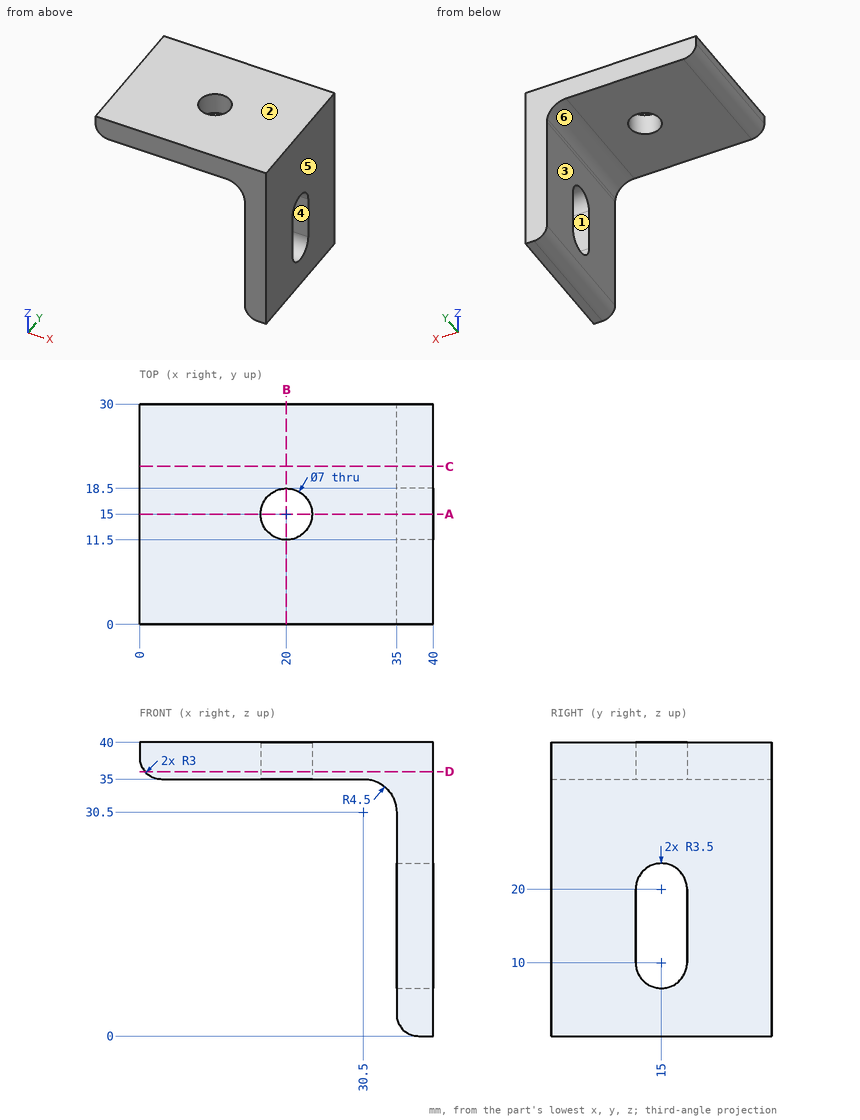
The figure shows three views and two pictorial views of one solid part (mm, origin at its lowest corner). Answer the questions. A direction names the side the tool comes from. Give positions to 0.01 mm unless a question says otherwise; leave off trailing zeros. Order: outer loops, then holes, each group sorted by start corner. A loop starts at its lowest first (then second) coordinate and runs counter-clockwise, first axis right, second up. Notation, with made-up numbers: (57, 13.5) -> (75, 13.5) arc R17 cw to (75, 43.5) -> close; hole circle Ø6 at (34.5, 75). An arc over 180 degrees is marked (long way). One line per item, written item: value.
1) Find section A-A, the plane y = 15. Determine the outline of the cut face in (x, z).
Reported:
outline: (0, 38) arc R3 ccw to (3, 35) -> (16.5, 35) -> (16.5, 40) -> (0, 40) -> close; (23.5, 35) -> (30.5, 35) arc R4.5 cw to (34.93, 31.3) arc R4.5 cw to (35, 30.5) -> (35, 23.5) -> (40, 23.5) -> (40, 40) -> (23.5, 40) -> close; (35, 3) arc R3 ccw to (38, 0) -> (40, 0) -> (40, 6.5) -> (35, 6.5) -> close
2) Find section D-D, the plane z = 36. Determine the outline of the cut face in (x, y), plus the area to 3 significant figures.
Reported:
outline: (0.76, 0) -> (40, 0) -> (40, 30) -> (0.76, 30) -> close; hole circle Ø7 at (20, 15)
area: 1,140 mm^2
3) Determine the mould class of the marked faces 4, 5 and 6 for opening direction Z: pulls with the +Z half, pulls with the -Z half, needs draft (parallel to the pull), parting line crosses it, or undercut.
Reported:
face 4: undercut
face 5: needs draft
face 6: pulls with the -Z half
4) Find section B-B, the plane x = 20. Determine the outline of the cut face in (y, z), plus the area to 3 significant figures.
Reported:
outline: (0, 35) -> (11.5, 35) -> (11.5, 40) -> (0, 40) -> close; (18.5, 35) -> (30, 35) -> (30, 40) -> (18.5, 40) -> close
area: 115 mm^2
5) Find section C-C, the plane y = 21.5. Determine the outline of the cut face in (x, z).
Reported:
outline: (0, 38) arc R3 ccw to (3, 35) -> (30.5, 35) arc R4.5 cw to (34.93, 31.3) arc R4.5 cw to (35, 30.5) -> (35, 3) arc R3 ccw to (38, 0) -> (40, 0) -> (40, 40) -> (0, 40) -> close
6) A tool of negligible diameter and unlimited length cuts with its end or side. For the marked faces 1, 2 and 3, from which of +Z, -Z, +X, -X, +Y, -Y can it reach the whole face along a straight path? Write none if from no direction.
Reported:
face 1: +X, -X
face 2: +Z, +X, -X, +Y, -Y
face 3: -Z, -X, +Y, -Y
7) Flat-ended cylindrical pins translate along their axes: P1, Ø10, axis at x = 35.5, z = 12, coming from the -Y side; P2, Ø10, axis at y = 6.5, z = 19.5, coming from the -X side; P3, Ø2, axis at x = 32.5, y = 10, coming from the -Z side. Find the tip coordinate at first contact, or state that the pin passes through.
Reported:
P1: stops at y = 0
P2: stops at x = 35
P3: stops at z = 33.85
8) Find the intervals of material crossed by line 1 (Y direction, x = 20, z = 38.05); line 2 (X direction, y = 16.25, z = 28.5); line 3 (Z direction, x = 36, y = 16.5), in increasing order.
Reported:
line 1: y = 0 to 11.5, 18.5 to 30
line 2: x = 35 to 40
line 3: z = 0.76 to 6.84, 23.16 to 40
